Source: CAD feature listing. Evaluate the final solid. Frame: model axes, mm. A direction names the side the tool comes from. Coordinates: 2 decimals unless noted, no trailing zeros. Write each loop counter-clockwise with the first axis right and the second up, starting at its lowest first coordinate (ties: lowest second). Pieces come first, ordered by that corner, then holes. Notation, with made-up numbers: (51.5, 67.25) -> (58.5, 67.25) arc R28 ccw to (58.5, 98.25) -> close; hole circle Ø9 at (-2.75, -36.75). An arc over 180 degrees is marked (long way). Write item = value, one per line.
from build123d import *

# Parameters (mm, degrees)
SKETCH1_R               = 37.5
SKETCH1_R_2             = 34
BOSS_EXTRUDE1_DEPTH     = 20
SKETCH2_R               = 37.5
BOSS_EXTRUDE2_DEPTH     = 3
SKETCH3_W               = 11
SKETCH3_H               = 25
CUT_EXTRUDE1_DEPTH      = 3
SKETCH4_R               = 1.5
CUT_EXTRUDE2_DEPTH      = 80
CUT_EXTRUDE2_DEPTH_BACK = 80
SKETCH5_R               = 1.5
CUT_EXTRUDE4_DEPTH      = 80
CUT_EXTRUDE4_DEPTH_BACK = 80


with BuildPart() as part:
    # Sketch1 → Boss-Extrude1 (new body)
    with BuildSketch(Plane(origin=(0, 0, 0), x_dir=(1, 0, 0), z_dir=(0, 1, 0))):
        Circle(SKETCH1_R)
        Circle(SKETCH1_R_2, mode=Mode.SUBTRACT)
    extrude(amount=BOSS_EXTRUDE1_DEPTH)

    # Sketch2 → Boss-Extrude2 (add)
    with BuildSketch(Plane(origin=(0, 20, 0), x_dir=(1, 0, 0), z_dir=(0, 1, 0))):
        Circle(SKETCH2_R)
    extrude(amount=BOSS_EXTRUDE2_DEPTH)

    # Sketch3 → Cut-Extrude1 (cut)
    with BuildSketch(Plane(origin=(0, 23, 0), x_dir=(1, 0, 0), z_dir=(0, 1, 0))):
        with Locations((26.118823508, 0)):
            Rectangle(SKETCH3_W, SKETCH3_H)
    extrude(amount=-CUT_EXTRUDE1_DEPTH, mode=Mode.SUBTRACT)

    # Sketch4 → Cut-Extrude2 (cut, two sides)
    with BuildSketch(Plane.XY) as cut_extrude2_sk:
        with Locations((0, 11.5)):
            Circle(SKETCH4_R)
    extrude(amount=CUT_EXTRUDE2_DEPTH, mode=Mode.SUBTRACT)
    extrude(cut_extrude2_sk.sketch, amount=-CUT_EXTRUDE2_DEPTH_BACK, mode=Mode.SUBTRACT)

    # Sketch5 → Cut-Extrude4 (cut, two sides)
    with BuildSketch(Plane(origin=(0, 0, 0), x_dir=(0, 0, -1), z_dir=(1, 0, 0))) as cut_extrude4_sk:
        with Locations((0, 11.5)):
            Circle(SKETCH5_R)
    extrude(amount=CUT_EXTRUDE4_DEPTH, mode=Mode.SUBTRACT)
    extrude(cut_extrude4_sk.sketch, amount=-CUT_EXTRUDE4_DEPTH_BACK, mode=Mode.SUBTRACT)


solid = part.part
1) Material intervals for probe 1 along Y at (x, z) = (-31.5, 11.5); probe 2 along Y at (x, z) = (0, 36); probe 3 along Z at (x, y) = (7.5, 18.25), sorted ascending. Write a range as [from, to].
Answer block:
probe_1 = [20, 23]
probe_2 = [0, 10], [13, 23]
probe_3 = [-36.74, -33.16], [33.16, 36.74]
2) First-contact query: pin 1 Ø2.5 at (y, z) = (21.5, -5) entering from +X; pin 2 Ø2.5 at (y, z) = (21, -5) entering from -X; pin 3 Ø2.5 at (x, y) = (25.5, 21.5) entering from +Z; pin 4 Ø2.5 at (y, z) = (11.5, 0) entering from -X. Flat tips, straight axial feed; report the tip coordinate or a pass-through.
Answer block:
pin_1 = 37.31
pin_2 = -37.31
pin_3 = 28.6
pin_4 = through
3) Cut plane A-A, the plane z = 0. Output: boundary loops of the cut face in (x, y).
Answer block:
outline = (-37.5, 0) -> (-34, 0) -> (-34, 10) -> (-37.5, 10) -> close; (-37.5, 13) -> (-34, 13) -> (-34, 20) -> (20.62, 20) -> (20.62, 23) -> (-37.5, 23) -> close; (31.62, 20) -> (34, 20) -> (34, 13) -> (37.5, 13) -> (37.5, 23) -> (31.62, 23) -> close; (34, 0) -> (37.5, 0) -> (37.5, 10) -> (34, 10) -> close
4) Reachability of faces 4 (the cylindrical face through (36, 10, 0)), 5 (the flat face through (26, 22, -12.5)), 6 (the flat face through (33, 20, 0)) from +Z, -Z, +X, -X, +Y, -Y: full face, straight path, thin tool, end or side. Return the list, or none.
Answer block:
face_4 = +X, -X
face_5 = +Y, -Y
face_6 = -Y
5) Cut plane D-D, the plane y = 11.5. Output: boundary loops of the cut face in (x, z).
Answer block:
outline = (-37.47, -1.5) arc R37.5 ccw to (-1.5, -37.47) -> (-1.5, -33.97) arc R34 cw to (-33.97, -1.5) -> close; (-37.47, 1.5) -> (-33.97, 1.5) arc R34 cw to (-1.5, 33.97) -> (-1.5, 37.47) arc R37.5 ccw to start; (1.5, -37.47) arc R37.5 ccw to (37.47, -1.5) -> (33.97, -1.5) arc R34 cw to (1.5, -33.97) -> close; (1.5, 33.97) arc R34 cw to (33.97, 1.5) -> (37.47, 1.5) arc R37.5 ccw to (1.5, 37.47) -> close
6) Pull-direction query (Y, two-part tool) for faces 1 (the cylindrical face through (0, 10, -36)), 2 (the flat face through (26, 22, 12.5)), 3 (the flat face through (8.2, 0, 33.2)); classes: +Y half, -Y half, draft (parallel to the pull), parting line (faces both ways), or undercut.
Answer block:
face_1 = undercut
face_2 = draft
face_3 = -Y half
7) Cut plane C-C, the plane x = 0. Output: boundary loops of the cut face in (y, z), and give its area (3 significant figures).
Answer block:
outline = (0, -37.5) -> (10, -37.5) -> (10, -34) -> (0, -34) -> close; (0, 34) -> (10, 34) -> (10, 37.5) -> (0, 37.5) -> close; (13, -37.5) -> (23, -37.5) -> (23, 37.5) -> (13, 37.5) -> (13, 34) -> (20, 34) -> (20, -34) -> (13, -34) -> close
area = 344 mm2
8) Cut plane B-B, the plane x = 30. Output: boundary loops of the cut face in (y, z), and give its area (3 significant figures).
Answer block:
outline = (0, -22.5) -> (23, -22.5) -> (23, -12.5) -> (20, -12.5) -> (20, -16) -> (0, -16) -> close; (0, 16) -> (20, 16) -> (20, 12.5) -> (23, 12.5) -> (23, 22.5) -> (0, 22.5) -> close
area = 320 mm2
